Work out the finished part from the listing and answer in its coordinate system (mm). Face numbers are marked on the shaded views. A direction names the side the tool comes from. Coordinates: 2 decimals unless noted, no trailing zeros. Write each loop counter-clockwise with the first axis right and the second up, starting at its lowest first coordinate (ties: lowest second). Pieces come first, ordered by that corner, then holes. Notation, with made-up numbers: (23.25, 23.25) - (47.25, 23.25) arc R33 ccw to (47.25, 57.25) - close; hole circle Ø2 at (-14.75, 60.25). An arc over 180 degrees is marked (long way). Answer as a JSON object with one key per item and string values. Group by question number.
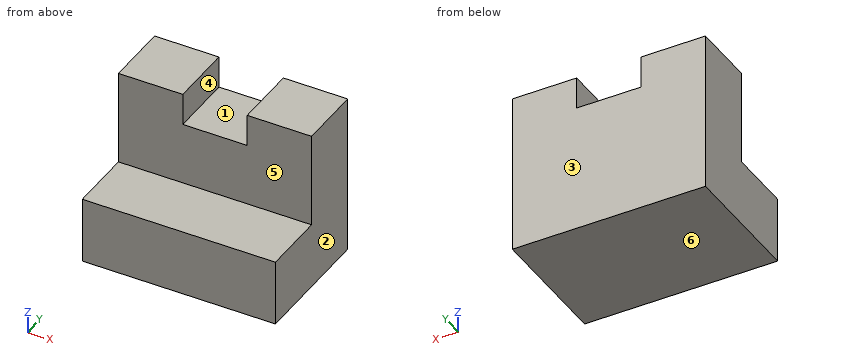
from build123d import *

# Parameters (mm, degrees)
F1_DEPTH = 25.4
F4_DEPTH = 12.7
F5_W     = 38.1
F5_H     = 13.0556984428
F6_DEPTH = 12.7


with BuildPart() as f1:
    # F0 (on Front) → F1 (new body)
    with BuildSketch(Plane.XZ):
        Polygon((-47.2752685128, 40.980277073), (-59.9752685128, 40.980277073), (-59.9752685128, 9.230277073), (-21.8752685128, 9.230277073), (-21.8752685128, 40.980277073), (-34.5752685128, 40.980277073), (-34.5752685128, 34.630277073), (-47.2752685128, 34.630277073), align=None)
    extrude(amount=F1_DEPTH)

    # F4 (cut): a face of the model
    f4_faces = [f1.faces().sort_by_distance(p)[0] for p in [
        (-40.9252685128, -25.4, 24.1981342159),
    ]]
    extrude(f4_faces, amount=-F4_DEPTH, mode=Mode.SUBTRACT)

    # F5 (on face) → F6 (join)
    with BuildSketch(Plane.XZ.offset(12.7)):
        with Locations((-40.9252685128, 15.7581262944)):
            Rectangle(F5_W, F5_H)
    extrude(amount=F6_DEPTH)


solid = f1.part
Q1. Consider L1, parallel to Z at x = -50.5, y = -19.5; L2, parallel to X at y = -11.5, z = 38; L3, parallel to Y at x = -48.5, z = 31. Determine where each line is inside the solid, lowest interval first. Write a range as from..to.
Q2. Section A-A on z = 36 is taken. Determine the outline of the cut face in (x, y).
Q3. Section B-B on y = -8.5 is taken. Determine the outline of the cut face in (x, z).
Q4. Section D-D on x = -44.5 is taken. Determine the outline of the cut face in (y, z).
Q5. Flat-ended cylindrical pins translate along their axes: pin 1 Ø5.5 at (x, z) = (-43, 27.5) entering from -Y; pin 2 Ø10 at (x, y) = (-32.5, -22) entering from +Z; pin 3 Ø4 at (x, y) = (-42, -5) entering from +Z. Find the tip coordinate at first contact, or state that the pin passes through.
Q6. For a pull along X with two mould halves and no side action, classify the marked faces 1, 2, 3 and 4 as +X half, -X half, draft (parallel to the pull), parting line (faces both ways), or undercut.
Q7. A tool of negligible diameter and unlimited length cuts with its end or side. For the marked faces 5 and 6, from which of +Z, -Z, +X, -X, +Y, -Y can it reach the whole face along a straight path? Write none if from no direction.
Q8. Section C-C on x = -49.5 is taken. Determine the outline of the cut face in (y, z).
Numbers:
{
 "1": {"L1": "z = 9.23..22.29", "L2": "x = -59.98..-47.28, -34.58..-21.88", "L3": "y = -12.7..0"},
 "2": {"outline": "(-59.98, -12.7) - (-47.28, -12.7) - (-47.28, 0) - (-59.98, 0) - close; (-34.58, -12.7) - (-21.88, -12.7) - (-21.88, 0) - (-34.58, 0) - close"},
 "3": {"outline": "(-59.98, 9.23) - (-21.88, 9.23) - (-21.88, 40.98) - (-34.58, 40.98) - (-34.58, 34.63) - (-47.28, 34.63) - (-47.28, 40.98) - (-59.98, 40.98) - close"},
 "4": {"outline": "(-25.4, 9.23) - (0, 9.23) - (0, 34.63) - (-12.7, 34.63) - (-12.7, 22.29) - (-25.4, 22.29) - close"},
 "5": {"pin 1": "stops at y = -12.7", "pin 2": "stops at z = 22.29", "pin 3": "stops at z = 34.63"},
 "6": {"face 1": "undercut", "face 2": "+X half", "face 3": "draft", "face 4": "undercut"},
 "7": {"face 5": "+Z, +X, -X, -Y", "face 6": "-Z, +X, -X, +Y, -Y"},
 "8": {"outline": "(-25.4, 9.23) - (0, 9.23) - (0, 40.98) - (-12.7, 40.98) - (-12.7, 22.29) - (-25.4, 22.29) - close"}
}
